Part model, mm, in its own coordinate system. A direction names the side the tool comes from. Coordinates: 2 decimals unless noted, no trailing zeros. Loops run counter-clockwise (first coordinate to the right, second up) from the corner with the lowest first, then second, coordinate; pieces in that order, holes last. Notation, with made-up numbers: (24, -38.5) -> (40, -38.5) arc R32 ccw to (40, -2.5) -> close; hole circle Ø8 at (20.5, 2). An arc over 180 degrees is marked (long way). Use one line per item in the form item = value. Start each with the question number.
(1) Drill centre lines: L1, parallel to Y at x = -389.75, z = 76.2 (3 decimals); L2, parallel to Z at x = -161.5, y = 15.5; L3, parallel to Z at x = -17, y = 120. Where is each one in solid material? Low to high. Write a range as [from, to].
(2) Mould opens along Y. For faces 1 (the flat face through (-205, 0, 75)), 2 (the cylindrical face through (-12.522, 126.946, 77.027)), 3 (the flat face through (-25.4, 84, 77)), 4 (the cylindrical face through (-391.338, 116.4, 70.657)) say: +Y half, -Y half, draft (parallel to the pull), parting line (faces both ways), or undercut.
(3) Band-saw the part on D-D on z = 12.7. Give the cut face in (x, y) (3 decimals), then the cut area to 3 significant figures.
(4) 3-axis set-ups, long thin cutter, end or side, ignore diameter. For faces 5 (the flat face through (0, 75, 75)), 6 (the flat face through (-204, 12.7, 75)): which of +Z, -Z, +X, -X, +Y, -Y reach the whole face in a straight line?
(5) Pin check, flat tips, straight feed: P1, Ø1, axis at x = -307.5, y = 102, coming from the -Z side; P2, Ø4, axis at x = -289.5, z = 128.5, coming from the +Y side. Stop position of each tip, or through.
(6) Band-saw the part on A-A on y = 120.65. Give the cut face in (x, z) (3 decimals).
(7) Band-saw the part on C-C on y = 62. Give the cut face in (x, z), then the cut area to 3 significant figures.
(8) Band-saw the part on B-B on z = 76.2. Give the cut face in (x, y) (3 decimals).
```python
from build123d import *

# Parameters (mm, degrees)
SKETCH1_W           = 403.86
SKETCH1_H           = 152.4
BOSS_EXTRUDE1_DEPTH = 152.4
SKETCH3_W           = 353.06
SKETCH3_H           = 101.6
CUT_EXTRUDE1_DEPTH  = 139.7
SKETCH4_R           = 5.715
BOSS_EXTRUDE2_DEPTH = 63.5
SKETCH5_R           = 6.35
CUT_EXTRUDE2_DEPTH  = 63.5
CUT_EXTRUDE3_REACH  = 405.86
SKETCH6_R           = 6.985
SKETCH7_R           = 5.715
BOSS_EXTRUDE3_DEPTH = 63.5


with BuildPart() as part:
    # Sketch1 → Boss-Extrude1 (new body)
    with BuildSketch(Plane.XY):
        with Locations((-201.93, 76.2)):
            Rectangle(SKETCH1_W, SKETCH1_H)
    extrude(amount=BOSS_EXTRUDE1_DEPTH)

    # Sketch3 → Cut-Extrude1 (cut)
    with BuildSketch(Plane(origin=(0, 152.4, 0), x_dir=(1, 0, 0), z_dir=(0, 1, 0))):
        with Locations((-201.93, -76.2)):
            Rectangle(SKETCH3_W, SKETCH3_H)
    extrude(amount=-CUT_EXTRUDE1_DEPTH, mode=Mode.SUBTRACT)

    # Sketch4 → Boss-Extrude2 (add)
    with BuildSketch(Plane(origin=(0, 152.4, 0), x_dir=(1, 0, 0), z_dir=(0, 1, 0))):
        with Locations((-391.16, -139.7)):
            Circle(SKETCH4_R)
    extrude(amount=BOSS_EXTRUDE2_DEPTH)

    # Sketch5 → Cut-Extrude2 (cut)
    with BuildSketch(Plane(origin=(0, 0, 0), x_dir=(0, 0, -1), z_dir=(1, 0, 0))):
        with Locations((-76.2, 120.65)):
            Circle(SKETCH5_R)
    extrude(amount=-CUT_EXTRUDE2_DEPTH, mode=Mode.SUBTRACT)

    # Sketch6 → Cut-Extrude3 (cut, up to next)
    with BuildSketch(Plane.ZY.offset(403.86), mode=Mode.PRIVATE) as cut_extrude3_sk1:
        with Locations((76.2, 120.65)):
            Circle(SKETCH6_R)
    cut_extrude3_tool1 = extrude(cut_extrude3_sk1.sketch, amount=-CUT_EXTRUDE3_REACH, mode=Mode.PRIVATE) & part.part
    add(cut_extrude3_tool1.solids().sort_by_distance((-403.86, 120.65, 76.2))[0], mode=Mode.SUBTRACT)

    # Sketch7 → Boss-Extrude3 (add)
    with BuildSketch(Plane(origin=(0, 152.4, 0), x_dir=(1, 0, 0), z_dir=(0, 1, 0))):
        with Locations((-12.7, -12.7)):
            Circle(SKETCH7_R)
    extrude(amount=BOSS_EXTRUDE3_DEPTH)


solid = part.part
```
A:
q1.L1 = [0, 113.665], [127.635, 152.4]
q1.L2 = [0, 25.4], [127, 152.4]
q1.L3 = [0, 69.88], [82.52, 152.4]
q2.face_1 = -Y half
q2.face_2 = undercut
q2.face_3 = draft
q2.face_4 = undercut
q3.outline = (-403.86, 0) -> (0, 0) -> (0, 152.4) -> (-6.985, 152.4) -> (-6.985, 215.9) -> (-18.415, 215.9) -> (-18.415, 152.4) -> (-403.86, 152.4) -> close
q3.area = 62,300 mm²
q4.face_5 = +Z, -Z, +X, +Y, -Y
q4.face_6 = +Y
q5.P1 = 0
q5.P2 = 152.4
q6.outline = (-403.86, 0) -> (0, 0) -> (0, 69.85) -> (-25.4, 69.85) -> (-25.4, 25.4) -> (-378.46, 25.4) -> (-378.46, 69.215) -> (-403.86, 69.215) -> close; (-403.86, 83.185) -> (-378.46, 83.185) -> (-378.46, 127) -> (-25.4, 127) -> (-25.4, 82.55) -> (0, 82.55) -> (0, 152.4) -> (-403.86, 152.4) -> close
q7.outline = (-403.86, 0) -> (0, 0) -> (0, 152.4) -> (-403.86, 152.4) -> close; hole (-378.46, 25.4) -> (-25.4, 25.4) -> (-25.4, 127) -> (-378.46, 127) -> close
q7.area = 25,700 mm²
q8.outline = (-403.86, 0) -> (0, 0) -> (0, 114.3) -> (-25.4, 114.3) -> (-25.4, 12.7) -> (-378.46, 12.7) -> (-378.46, 113.665) -> (-403.86, 113.665) -> close; (-403.86, 127.635) -> (-378.46, 127.635) -> (-378.46, 152.4) -> (-403.86, 152.4) -> close; (-25.4, 127) -> (0, 127) -> (0, 152.4) -> (-25.4, 152.4) -> close
